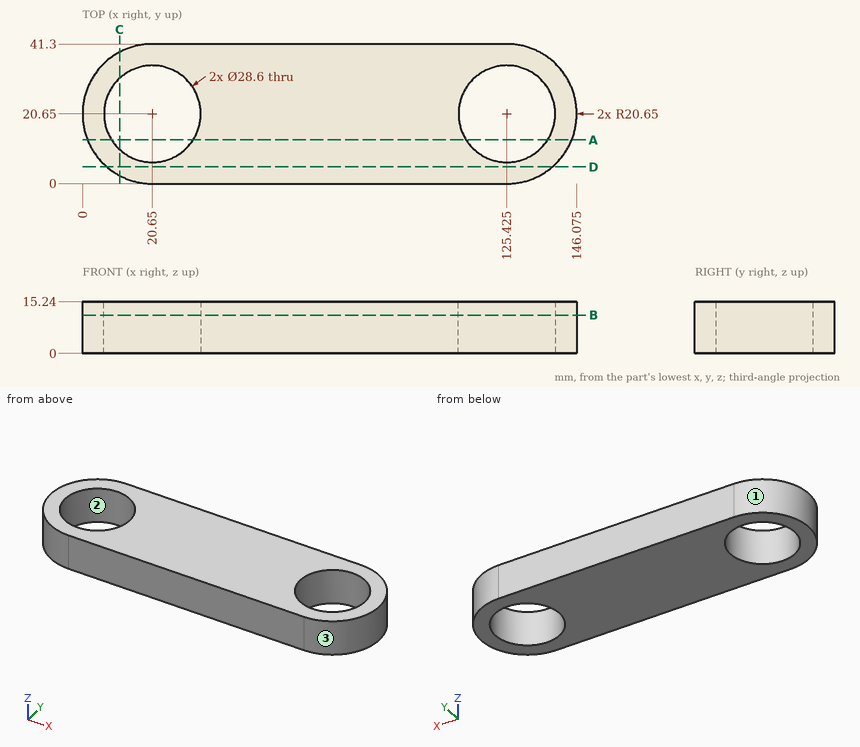
For this review, use the dimensioned drawing (mm, ordinates from the lowest corner) and the shaded views. Round coordinates to 2 decimals unless told otherwise and drop trailing zeros. Write each loop counter-clockwise with the first axis right and the second up, starting at its lowest first coordinate (ties: lowest second). Pieces come first, ordered by that corner, then holes. Notation, with made-up numbers: (51, 33) -> (89, 33) arc R21 cw to (89, 60) -> close; hole circle Ø8 at (1.25, -17). An arc over 180 degrees is marked (long way). Use one line per item in the form item = value.
Q1. Consider section C-C (x = 11). State the section outline as (y, z) points.
Resolved:
outline = (2.39, 0) -> (10.1, 0) -> (10.1, 15.24) -> (2.39, 15.24) -> close; (31.2, 0) -> (38.91, 0) -> (38.91, 15.24) -> (31.2, 15.24) -> close
Q2. Consider section D-D (y = 5). State the section outline as (x, z) points.
Resolved:
outline = (7.18, 0) -> (138.9, 0) -> (138.9, 15.24) -> (7.18, 15.24) -> close
Q3. The part is to be moulded in two halves that separate along X. For the marked faces 1, 2 and 3, say which applies: released by +X, released by -X, zero draft, split by the parting line, or undercut.
Resolved:
face_1 = released by -X
face_2 = undercut
face_3 = released by +X
Q4. Clearance check with flat-ended pins moving along their axes: pin 1 Ø3 at (x, y) = (76, 36) entering from -Z; pin 2 Ø3 at (y, z) = (15, 4.5) entering from +X; pin 3 Ø6 at (x, z) = (14.5, 10) entering from +Y; pin 4 Ø8 at (y, z) = (7.5, 12.5) entering from +X. State where each tip first meets the part, or that it passes through.
Resolved:
pin_1 = 0
pin_2 = 145.65
pin_3 = 41.06
pin_4 = 143.94
Q5. To check wall thickness, follow probe 1 along X at (y, z) = (25, 2.25); probe 2 along X at (y, z) = (27.5, 8) (1 decimal); probe 3 along Y at (x, z) = (114, 9.75). State the ranges of each line that lie inside material, in increasing order. Write a range as from..to.
Resolved:
probe_1 = 0.46..7.03, 34.27..111.8, 139.05..145.61
probe_2 = 1.2..8.1, 33.2..112.9, 138..144.9
probe_3 = 0..12.05, 29.25..41.3
Q6. Consider section B-B (z = 11.25). State how many separate pieces and enclosed holes the cut face has, then the cut area to 3 significant figures.
Resolved:
separate_pieces = 1
enclosed_holes = 2
area = 4,380 mm²
Q7. Consider section A-A (y = 13). State the section outline as (x, z) points.
Resolved:
outline = (1.47, 0) -> (8.57, 0) -> (8.57, 15.24) -> (1.47, 15.24) -> close; (32.73, 0) -> (113.34, 0) -> (113.34, 15.24) -> (32.73, 15.24) -> close; (137.51, 0) -> (144.61, 0) -> (144.61, 15.24) -> (137.51, 15.24) -> close
